Verification items for the finished model (mm, model axes). Coordinates: 2 decimals unless noted, no trailing zeros. Loops run counter-clockwise (first coordinate to the right, second up) from the corner with the lowest first, then second, coordinate; pieces in that order, holes last.
Q1. Sectioned sample at C-C (z = -1.5). Enter the section's corners in (x, y), then the cut area to 3 significant figures.
Q2. Sectioned sample at D-D (z = 37). Enter the section's corners in (x, y), then the cut area to 3 significant figures.
Q3. Go/stop test with a flat-tipped pin: P1, Ø2, axis at y = 4, z = -8, coming from the +X side. Record where the tip stops, or that it passes through.
Q4. Material ranges on probe 1 along X at (y, z) = (1.5, 0); probe 2 along X at (y, z) = (2, 40); probe 3 along Z at (x, y) = (3, 4.75), recorded low to high.
Q5. Mould release check, pull along Z, two halves, no side actions. Record for faces 1 (the face through (6.35, 3, 52)), 2 (the face through (5.037, 3.131, 0.661)), 3 (the face through (13, 3, 86.36)), 4 (the face through (-15.156, 3.131, -11.542)): +Z half, -Z half, draft (parallel to the pull), parting line (faces both ways), or undercut.
Q6. Sectioned sample at B-B (y = 3). Enter the section's corners in (x, z), then the cut area to 3 significant figures.
Q7. Sectioned sample at A-A (x = 0). Enter the section's corners in (y, z), then the cut area to 3 significant figures.
```python
from build123d import *

# Parameters (mm, degrees)
SKETCH1_R           = 19.05
BOSS_EXTRUDE1_DEPTH = 6.35
SKETCH2_W           = 12.7
SKETCH2_H           = 86.36
BOSS_EXTRUDE2_DEPTH = 6.35
SKETCH3_R           = 5.08
CUT_EXTRUDE1_DEPTH  = 6.35


with BuildPart() as part:
    # Sketch1 → Boss-Extrude1 (new body)
    with BuildSketch(Plane(origin=(0, 0, 0), x_dir=(1, 0, 0), z_dir=(0, 1, 0))):
        with Locations(Location((0, 0, 0), (0, 0, 270))):
            Circle(SKETCH1_R)
    extrude(amount=BOSS_EXTRUDE1_DEPTH)

    # Sketch2 → Boss-Extrude2 (add)
    with BuildSketch(Plane.XZ):
        with Locations((12.7, 43.18)):
            Rectangle(SKETCH2_W, SKETCH2_H)
    extrude(amount=-BOSS_EXTRUDE2_DEPTH)

    # Sketch3 → Cut-Extrude1 (cut)
    with BuildSketch(Plane.XZ):
        with Locations(Location((0, 0, 0), (0, 0, 270))):
            Circle(SKETCH3_R)
    extrude(amount=-CUT_EXTRUDE1_DEPTH, mode=Mode.SUBTRACT)


solid = part.part
```
Geometry check:
1. outline: (-18.99, 0) - (-4.85, 0) - (-4.85, 6.35) - (-18.99, 6.35) - close; (4.85, 0) - (18.99, 0) - (18.99, 6.35) - (4.85, 6.35) - close
1. area: 180 mm2
2. outline: (6.35, 0) - (19.05, 0) - (19.05, 6.35) - (6.35, 6.35) - close
2. area: 80.6 mm2
3. P1: stops at x = 17.72
4. probe 1: x = -19.05 to -5.08, 5.08 to 19.05
4. probe 2: x = 6.35 to 19.05
4. probe 3: z = -18.81 to -4.1, 4.1 to 18.81
5. face 1: draft
5. face 2: undercut
5. face 3: +Z half
5. face 4: parting line
6. outline: (6.35, 17.96) arc R19.05 ccw (long way) to (19.05, 0) - (19.05, 86.36) - (6.35, 86.36) - close; hole circle Ø10.16 at (0, 0)
6. area: 1,990 mm2
7. outline: (0, -19.05) - (6.35, -19.05) - (6.35, -5.08) - (0, -5.08) - close; (0, 5.08) - (6.35, 5.08) - (6.35, 19.05) - (0, 19.05) - close
7. area: 177 mm2
